Here's how the part is built. I have some questions about the finished solid (model axes, mm). A direction names the side the tool comes from. Coordinates: 2 decimals unless noted, no trailing zeros. Loops run counter-clockwise (first coordinate to the right, second up) from the corner with the lowest first, then second, coordinate; pieces in that order, holes last. Notation, with made-up numbers: (36.25, 15.5) -> (55.25, 15.5) arc R10 cw to (55.25, 28.5) -> close; hole circle Ø8 at (-32, -7). An arc over 180 degrees is marked (long way). Use CSV: the item, a comma, the result in double quotes. Start each with the question number.
from build123d import *

# Parameters (mm, degrees)
BOSS_EXTRUDE1_DEPTH = 6
SKETCH4_R           = 6
BOSS_EXTRUDE2_DEPTH = 6
SKETCH3_R           = 2
SKETCH3_R_2         = 6
CUT_EXTRUDE1_DEPTH  = 353.937671551


with BuildPart() as part:
    # Sketch2 → Boss-Extrude1 (new body)
    with BuildSketch(Plane(origin=(0, 0, 0), x_dir=(0, 0, -1), z_dir=(1, 0, 0))):
        Polygon((6, 352), (0, 352), (-25, 327), (-25, 25), (6, -6), align=None)
    extrude(amount=BOSS_EXTRUDE1_DEPTH)

    # Sketch4 → Boss-Extrude2 (add)
    with BuildSketch(Plane(origin=(6, 0, 0), x_dir=(0, 0, -1), z_dir=(1, 0, 0))):
        with Locations((-12, 340)):
            Circle(SKETCH4_R)
    extrude(amount=-BOSS_EXTRUDE2_DEPTH)

    # Sketch3 → Cut-Extrude1 (cut, through all)
    with BuildSketch(Plane(origin=(6, 0, 0), x_dir=(0, 0, -1), z_dir=(1, 0, 0))):
        with Locations((-12, 340)):
            Circle(SKETCH3_R)
        with Locations((-12, 12)):
            Circle(SKETCH3_R_2)
    extrude(amount=-CUT_EXTRUDE1_DEPTH, mode=Mode.SUBTRACT)


solid = part.part
1) Thinking about a two-plate mould opening in Z: for faces 3 (the face through (0, 176, 10)), 4 (the face through (3, 1, 1)), 5 (the face through (3, 348, 4)), which applies, pulls with the +Z half, pulls with the -Z half, needs draft (parallel to the pull), parting line crosses it, or undercut?
2) Please list where these lines run through material, in increasing order: L1, parallel to Y at x = 3.65, z = 12; L2, parallel to Z at x = 3.1, y = 340; L3, parallel to Y at x = 4.7, z = 6.5. Write a range as [from, to].
3) I want a section at A-A, the plane x = 1.3. Please give me the cut outline in (y, z).
4) I want a section at B-B, the plane y = 12. Please give me the cut outline in (x, z).
5) For P1, Ø2, axis at x = 5, z = 14.5, coming from the -Y side, with a flat end and sliding along its axis, tell me the tip position at first contact or that it passes through.
6) Which directions (+Z, -Z, +X, -X, +Y, -Y) give clear straight access to the entire face, cutting with the end or side of a thin tool? Please do faces 1 (the face through (3, 331, 21)), 2 (the face through (3, 178, 25)).
Return value:
1,face 3,"needs draft"
1,face 4,"pulls with the +Z half"
1,face 5,"undercut"
2,L1,"y = [18, 338], [342, 346]"
2,L2,"z = [-6, 10], [14, 18]"
2,L3,"y = [6.5, 9.6], [14.4, 345.5]"
3,outline,"(-6, -6) -> (352, -6) -> (352, 0) -> (344.24, 7.76) arc R6 ccw to (335.76, 16.24) -> (327, 25) -> (25, 25) -> (16.24, 16.24) arc R6 cw to (7.76, 7.76) -> close; hole circle Ø4 at (340, 12)"
4,outline,"(0, -6) -> (6, -6) -> (6, 6) -> (0, 6) -> close"
5,P1,"stops at y = 16.87"
6,face 1,"+Z, +X, -X"
6,face 2,"+Z, +X, -X, +Y, -Y"
